Can you work these out from the drawing? Everything is in mm from the part's minimum corner. Coordinates: 2 decimals unless noted, no trailing zeros. Order: outer loops, then holes, each group sorted by start corner. A loop starts at its lowest first (then second) coordinate and runs counter-clockwise, first axis right, second up. Notation, with made-up numbers: (44.25, 36) - (95.25, 36) arc R20 ccw to (95.25, 68) - close; hole circle Ø7 at (51, 61). An arc over 180 degrees is marked (long way). Answer as CSV lines item,"result". Start each with the question number.
Item 1: I need wall thicknesses on line 1 (X direction, y = 48.5, z = 5.5); line 2 (Y direction, x = 16.5, z = 6.75); line 3 (X direction, y = 115, z = 0.75). Which ranges of each line are inside material? Lowest first, please.
Item 2: I'm going to push flat-ended pins straight in: pin 1 (1.5 mm diameter, centred on y = 83.5, z = 2, fed in from -X); pin 2 (1.5 mm diameter, centred on x = 79, z = 9, fed in from -Y); pin 3 (1 mm diameter, centred on x = 23, z = 1.5, fed in from +Y). Where does each tip first touch, or does it pass through?
Item 3: Imagine slicing it at A-A on z = 6. List the corners of the cut face in (x, y) for me, and give its area (3 significant figures).
Item 4: Imagine slicing it at B-B on y = 20. List the corners of the cut face in (x, z) for me.
Item 5: Imagine slicing it at C-C on x = 74. List the corners of the cut face in (y, z) for me, and give its area (3 significant figures).
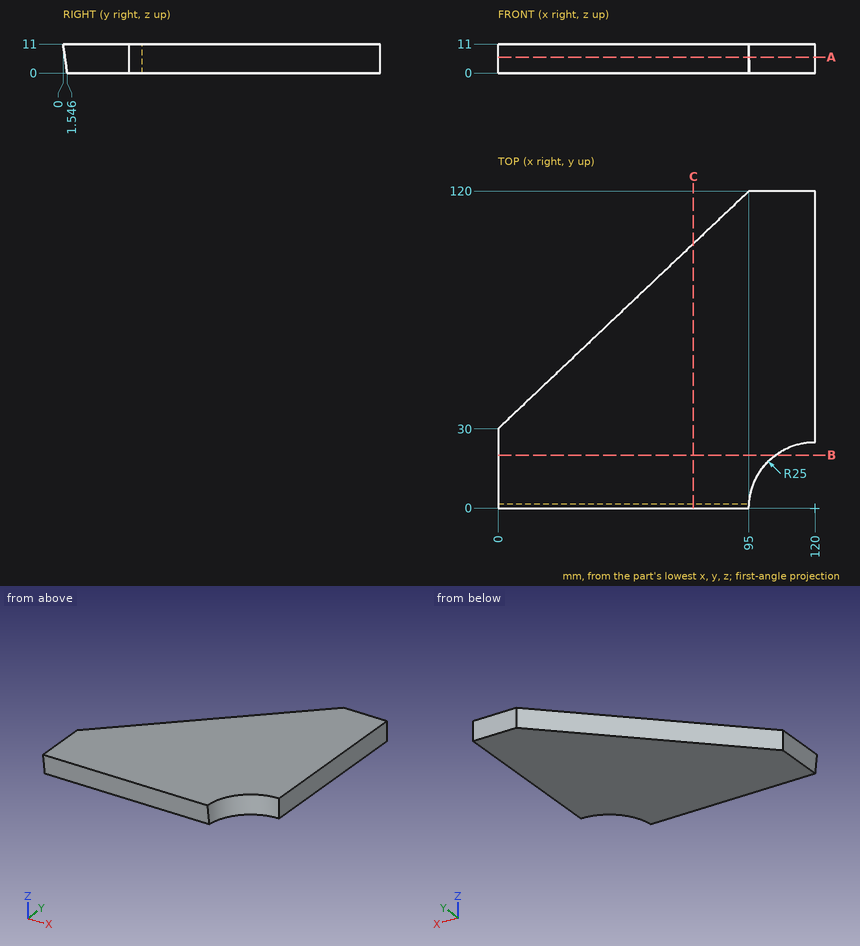
Responses:
1,line 1,"x = 19.53 to 120"
1,line 2,"y = 0.6 to 45.63"
1,line 3,"x = 89.72 to 120"
2,pin 1,"stops at x = 55.68"
2,pin 2,"stops at y = 0.18"
2,pin 3,"stops at y = 52.26"
3,outline,"(0, 0.7) - (95.01, 0.7) arc R25 cw to (120, 25) - (120, 120) - (95, 120) - (0, 30) - close"
3,area,"9,570 mm^2"
4,outline,"(0, 0) - (105, 0) - (105, 11) - (0, 11) - close"
5,outline,"(0, 11) - (1.55, 0) - (100.11, 0) - (100.11, 11) - close"
5,area,"1,090 mm^2"
